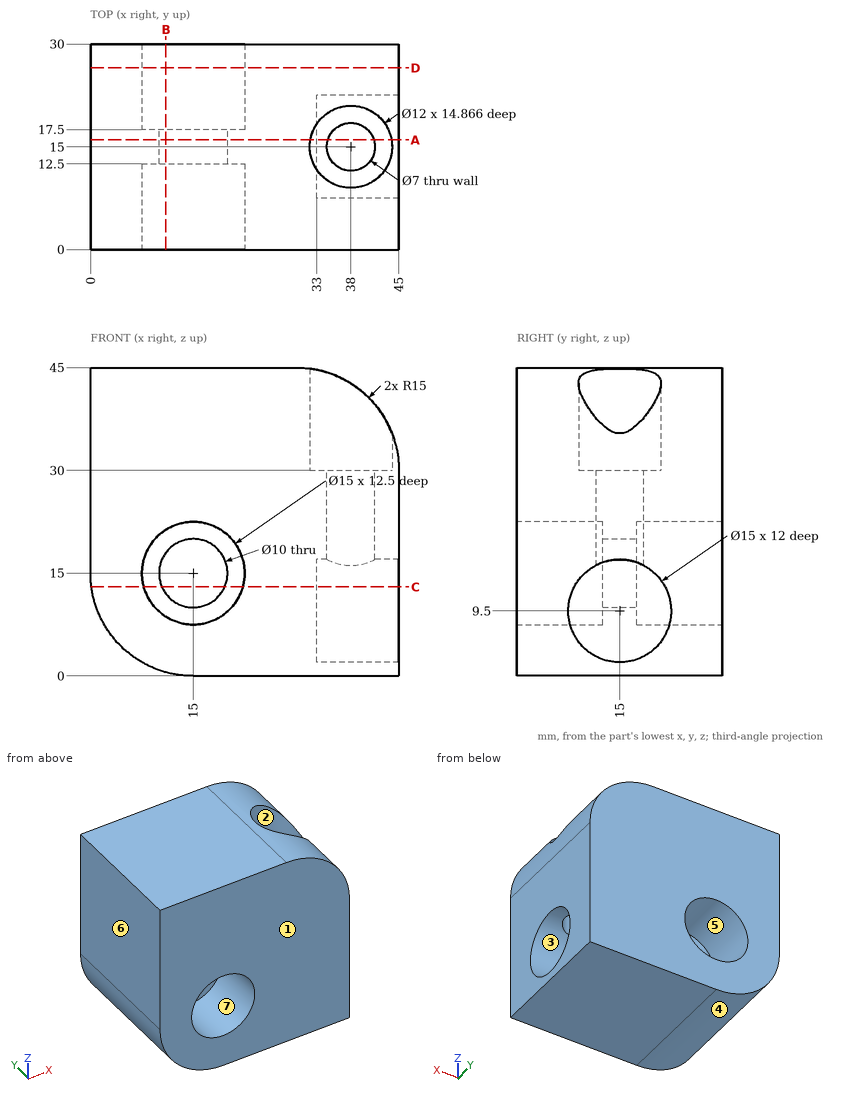
Part print with two shaded views. Sizes in mm from the minimum x, y, z corner. A direction names the side the tool comes from. Round coordinates to 2 decimals unless told otherwise and drop trailing zeros. Loops run counter-clockwise (first coordinate to the right, second up) from the corner with the lowest first, then second, coordinate; pieces in that order, holes last. Notation, with made-up numbers: M 56.5,79 L 106.5,79 A7 ccw 106.5,86 Z; hole C 3.25,29 d10. An arc over 180 degrees is marked long. Return JSON: item names as keys, results as strings. Group by question number.
(1) Drop flat-ended pins along their axis: P1, Ø11, axis at x = 38, y = 15, coming from the +Z side; P2, Ø11.5, axis at x = 15, z = 15, coming from the +Y side; P3, Ø3, axis at y = 25, z = 7, coming from the -X side. Give the stop position or say it passes through.
(2) Tool access for the marked faces 5, 6 and 7: list every direction of +Z, -Z, +X, -X, +Y, -Y with a clear straight run to the whole face (end or side of a thin tool).
(3) Saw through at A-A, the plane y = 16. List the corners of the cut face in (x, z), and give its area (3 significant figures).
(4) Mould opens along Y. For the marked faces 1, 2, 3 and 4 say: +Y half, -Y half, draft (parallel to the pull), parting line (faces both ways), or undercut.
(5) Saw through at B-B, the plane x = 11. List the corners of the cut face in (y, z).
(6) Saw through at D-D, the plane y = 26.5. List the corners of the cut face in (x, z).
(7) Saw through at C-C, the plane z = 13. List the corners of the cut face in (x, y).
(8) Wall check: probe 1 along X at (y, z) = (25.25, 15); probe 2 along Y at (x, z) = (38, 26.5); probe 3 along X at (y, z) = (15, 19). Give the ranges that are in metal, low to high. Write a range as [from, to].
Answer list:
{
 "1": {"P1": "z = 30", "P2": "y = 17.5", "P3": "x = 1.48"},
 "2": {"face 5": "+Y", "face 6": "+Z, -Z, -X, +Y, -Y", "face 7": "-Y"},
 "3": {"outline": "M 0,15 A15 ccw 15,0 L 45,0 L 45,2.07 L 33,2.07 L 33,16.93 L 34.65,16.93 L 34.65,30 L 32.08,30 L 32.08,44.85 A15 ccw 30,45 L 0,45 Z; M 41.35,16.93 L 45,16.93 L 45,30 A15 ccw 43.92,35.6 L 43.92,30 L 41.35,30 Z; hole C 15,15 d10", "area": "1,440 mm2"},
 "4": {"face 1": "-Y half", "face 2": "undercut", "face 3": "undercut", "face 4": "draft"},
 "5": {"outline": "M 0,0.54 L 30,0.54 L 30,8.66 L 17.5,8.66 L 17.5,12 L 12.5,12 L 12.5,8.66 L 0,8.66 Z; M 0,21.34 L 12.5,21.34 L 12.5,18 L 17.5,18 L 17.5,21.34 L 30,21.34 L 30,45 L 0,45 Z"},
 "6": {"outline": "M 0,15 A15 ccw 15,0 L 45,0 L 45,30 A15 ccw 30,45 L 0,45 Z; hole C 15,15 d15"},
 "7": {"outline": "M 0.13,0 L 7.77,0 L 7.77,12.5 L 10.42,12.5 L 10.42,17.5 L 7.77,17.5 L 7.77,30 L 0.13,30 Z; M 19.58,12.5 L 22.23,12.5 L 22.23,0 L 45,0 L 45,8.37 L 33,8.37 L 33,21.63 L 45,21.63 L 45,30 L 22.23,30 L 22.23,17.5 L 19.58,17.5 Z"},
 "8": {"probe 1": "[0, 7.5], [22.5, 45]", "probe 2": "[0, 11.5], [18.5, 30]", "probe 3": "[0, 12], [18, 34.5], [41.5, 45]"}
}
